```python
from build123d import *

# Parameters (mm, degrees)
F0_W     = 60
F0_H     = 80
F0_W_2   = 47
F0_H_2   = 66
F1_DEPTH = 60
F3_DEPTH = 60.001
F5_DEPTH = 80.001
F7_DEPTH = 10


with BuildPart() as f1:
    # F0 (on Top) → F1 (new body)
    with BuildSketch(Plane.XY):
        Rectangle(F0_W, F0_H)
        with Locations((-1.5, 3)):
            Rectangle(F0_W_2, F0_H_2, mode=Mode.SUBTRACT)
    extrude(amount=F1_DEPTH)

    # F2 (on face) → F3 (cut, through all)
    with BuildSketch(Plane.YZ.offset(30)):
        Polygon((-19.343146, 55), (-25, 49.343146), (-19.343146, 43.686292), (-13.686292, 49.343146), align=None)
        Polygon((-4.447715, 55), (-10.104569, 49.343146), (-4.447715, 43.686292), (1.209139, 49.343146), align=None)
        Polygon((10.447715, 55), (4.790861, 49.343146), (10.447715, 43.686292), (16.104569, 49.343146), align=None)
        Polygon((25.343146, 55), (19.686292, 49.343146), (25.343146, 43.686292), (31, 49.343146), align=None)
        Polygon((-10.104569, 30), (-4.447715, 24.343146), (1.209139, 30), (-4.447715, 35.656854), align=None)
        Polygon((25.343146, 24.343146), (31, 30), (25.343146, 35.656854), (19.686292, 30), align=None)
        Polygon((-19.343146, 35.656854), (-25, 30), (-19.343146, 24.343146), (-13.686292, 30), align=None)
        Polygon((10.447715, 35.656854), (4.790861, 30), (10.447715, 24.343146), (16.104569, 30), align=None)
        Polygon((-10.104569, 10.656854), (-4.447715, 5), (1.209139, 10.656854), (-4.447715, 16.313708), align=None)
        Polygon((25.343146, 5), (31, 10.656854), (25.343146, 16.313708), (19.686292, 10.656854), align=None)
        Polygon((-19.343146, 16.313708), (-25, 10.656854), (-19.343146, 5), (-13.686292, 10.656854), align=None)
        Polygon((10.447715, 16.313708), (4.790861, 10.656854), (10.447715, 5), (16.104569, 10.656854), align=None)
    extrude(amount=-F3_DEPTH, mode=Mode.SUBTRACT)

    # F4 (on face) → F5 (cut, through all)
    with BuildSketch(Plane(origin=(0, 40, 0), x_dir=(-1, 0, 0), z_dir=(0, 1, 0))):
        Polygon((-12.757359, 55), (-17, 50.757359), (-12.757359, 46.514719), (-8.514719, 50.757359), align=None)
        Polygon((-8.514719, 30), (-12.757359, 34.242641), (-17, 30), (-12.757359, 25.757359), align=None)
        Polygon((-8.514719, 9.242641), (-12.757359, 13.485281), (-17, 9.242641), (-12.757359, 5), align=None)
        Polygon((5.742641, 50.757359), (1.5, 55), (-2.742641, 50.757359), (1.5, 46.514719), align=None)
        Polygon((5.742641, 30), (1.5, 34.242641), (-2.742641, 30), (1.5, 25.757359), align=None)
        Polygon((5.742641, 9.242641), (1.5, 13.485281), (-2.742641, 9.242641), (1.5, 5), align=None)
        Polygon((20, 50.757359), (15.757359, 55), (11.514719, 50.757359), (15.757359, 46.514719), align=None)
        Polygon((20, 30), (15.757359, 34.242641), (11.514719, 30), (15.757359, 25.757359), align=None)
        Polygon((20, 9.242641), (15.757359, 13.485281), (11.514719, 9.242641), (15.757359, 5), align=None)
    extrude(amount=-F5_DEPTH, mode=Mode.SUBTRACT)

    # F6 (on Top) → F7 (join)
    with BuildSketch(Plane.XY):
        Polygon((0, 0), (60, -60), (60, 60), align=None)
        Polygon((-60, -60), (60, -60), (0, 0), align=None)
        Polygon((-60, 60), (-60, -60), (0, 0), align=None)
        Polygon((0, 0), (60, 60), (-60, 60), align=None)
    extrude(amount=-F7_DEPTH)


solid = f1.part
```
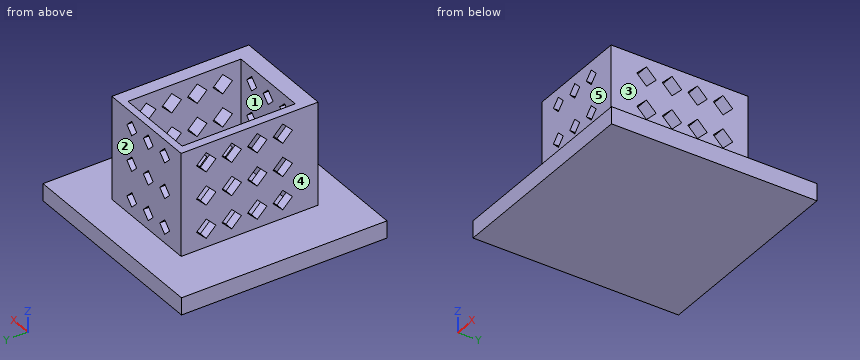
Source: CAD feature listing. Evaluate the final solid. Frame: model axes, mm. Face numbers are marked on the shaded views. A direction names the side the tool comes from. Round coordinates to 2 decimals unless told otherwise and drop trailing zeros. Loops run counter-clockwise (first coordinate to the right, second up) from the corner with the lowest first, then second, coordinate; pieces in that order, holes last. Notation, with made-up numbers: M 49.5,39 L 66.5,39 A9 ccw 66.5,51 Z; hole C 68,32 d5. An arc over 180 degrees is marked long. Use a Markdown table: item, result. Add a question column.
1. Section query A-A on z = 21. Return the cut outline in (x, y), then the cut area to 3 significant figures.
2. Section query D-D on x = 38. Return the cut outline in (y, z), then the cut area to 3 significant figures.
3. Contact query for flat-ended pins moving along their axis: P1, Ø6, axis at x = 22, z = 31, coming from the -Y side; P2, Ø14, axis at x = 9, z = 25, coming from the +Y side; P3, Ø1.5, axis at x = -9.5, y = 18, coming from the +Z side. Output: stop coordinate, or through.
4. Reachability of the marked faces 1, 2, 3, 4 and 5 from +Z, -Z, +X, -X, +Y, -Y: full face, straight path, thin tool, end or side. Return the list, or none.
5. Line query: line 1 (Y direction, x = -9, z = 41); line 2 (Y direction, x = -29.5, z = 12); line 3 (X direction, y = 12.5, z = 7). Output: solid intervals per line, ascending.
6. Section query B-B on y = -38. Give the number of separate pieces and of enclosed holes in the cut face, then the cut area to 3 significant figures.
Reported:
| question | item | result |
|---|---|---|
| 1 | outline | M -30,-40 L 30,-40 L 30,40 L -30,40 Z; hole M -25,-30 L 22,-30 L 22,36 L -25,36 Z |
| 1 | area | 1,700 mm² |
| 2 | outline | M -60,-10 L 60,-10 L 60,0 L -60,0 Z |
| 2 | area | 1,200 mm² |
| 3 | P1 | stops at y = -40 |
| 3 | P2 | stops at y = 40 |
| 3 | P3 | stops at z = 0 |
| 4 | face 1 | +Z |
| 4 | face 2 | +Z, +X, -X, +Y |
| 4 | face 3 | +Z, +X, +Y, -Y |
| 4 | face 4 | +Z, -X, +Y, -Y |
| 4 | face 5 | +Z, +X, -X, -Y |
| 5 | line 1 | y = -40 to -30, 36 to 40 |
| 5 | line 2 | y = -40 to -23.66, -15.03 to -8.76, -0.13 to 6.13, 14.76 to 21.03, 29.66 to 40 |
| 5 | line 3 | x = -30 to -25, 22 to 30 |
| 6 | separate pieces | 1 |
| 6 | enclosed holes | 9 |
| 6 | area | 4,480 mm² |
